```python
from build123d import *

# Parameters (mm, degrees)
EXTRUDE_1_DEPTH     = 3
EXTRUDE_2_DEPTH     = 51
EXTRUDE_3_DEPTH     = 3
FILLET_1_R          = 2
CHAMFER_1_SIZE      = 0.5
SKETCH_4_W          = 10
SKETCH_4_H          = 38
CUT_EXTRUDE_1_DEPTH = 59.180882402
FILLET_2_R          = 3


with BuildPart() as part:
    # 草图1 → 凸台-拉伸1 (new body)
    with BuildSketch(Plane.XY):
        with BuildLine():
            Line((-4, 1.5), (4, 1.5))
            ThreePointArc((4, 1.5), (5.5, 0), (4, -1.5))
            Line((4, -1.5), (-4, -1.5))
            ThreePointArc((-4, -1.5), (-5.5, 0), (-4, 1.5))
        make_face()
    extrude(amount=EXTRUDE_1_DEPTH)

    # 草图2 → 凸台-拉伸2 (add)
    with BuildSketch(Plane.XY.offset(3)):
        with BuildLine():
            Line((-10, 4.501256289), (-10, -1.5))
            Line((-10, -1.5), (-4, -1.5))
            ThreePointArc((-4, -1.5), (-5.5, 0), (-4, 1.5))
            Line((-4, 1.5), (4, 1.5))
            ThreePointArc((4, 1.5), (5.5, 0), (4, -1.5))
            Line((4, -1.5), (10, -1.5))
            Line((10, -1.5), (10, 4.501256289))
            ThreePointArc((10, 4.501256289), (0, 4), (-10, 4.501256289))
        make_face()
        with BuildLine():
            Line((4, 1.5), (-4, 1.5))
            ThreePointArc((-4, 1.5), (-5.5, 0), (-4, -1.5))
            Line((-4, -1.5), (4, -1.5))
            ThreePointArc((4, -1.5), (5.5, 0), (4, 1.5))
        make_face()
    extrude(amount=EXTRUDE_2_DEPTH)

    # 草图3 → 凸台-拉伸3 (add)
    with BuildSketch(Plane.XY.offset(54)):
        with BuildLine():
            Line((-3.954732622, 1.5), (4.045267378, 1.5))
            ThreePointArc((4.045267378, 1.5), (5.545267378, 0), (4.045267378, -1.5))
            Line((4.045267378, -1.5), (-3.954732622, -1.5))
            ThreePointArc((-3.954732622, -1.5), (-5.454732622, 0), (-3.954732622, 1.5))
        make_face()
    extrude(amount=EXTRUDE_3_DEPTH)

    # 圆角1
    fillet_1_edges = [part.edges().sort_by_distance(p)[0] for p in [
        (-10, -1.5, 28.5),
        (10, -1.5, 28.5),
    ]]
    fillet(fillet_1_edges, radius=FILLET_1_R)

    # 倒角1
    chamfer_1_edges = [part.edges().sort_by_distance(p)[0] for p in [
        (-5.454732622, 0, 57),
        (0.045267378, -1.5, 57),
        (5.545267378, 0, 57),
        (0.045267378, 1.5, 57),
        (0, 1.5, 0),
        (5.5, 0, 0),
        (0, -1.5, 0),
        (-5.5, 0, 0),
    ]]
    chamfer(chamfer_1_edges, length=CHAMFER_1_SIZE)

    # 草图4 → 切除-拉伸1 (cut, through all)
    with BuildSketch(Plane.XZ.offset(1.5)):
        with Locations((0, 28)):
            Rectangle(SKETCH_4_W, SKETCH_4_H)
    extrude(amount=-CUT_EXTRUDE_1_DEPTH, mode=Mode.SUBTRACT)

    # 圆角2
    fillet_2_edges = [part.edges().sort_by_distance(p)[0] for p in [
        (5, 1.312539111, 47),
        (5, 1.312539111, 9),
        (-5, 1.312539111, 9),
        (-5, 1.312539111, 47),
    ]]
    fillet(fillet_2_edges, radius=FILLET_2_R)


solid = part.part
```
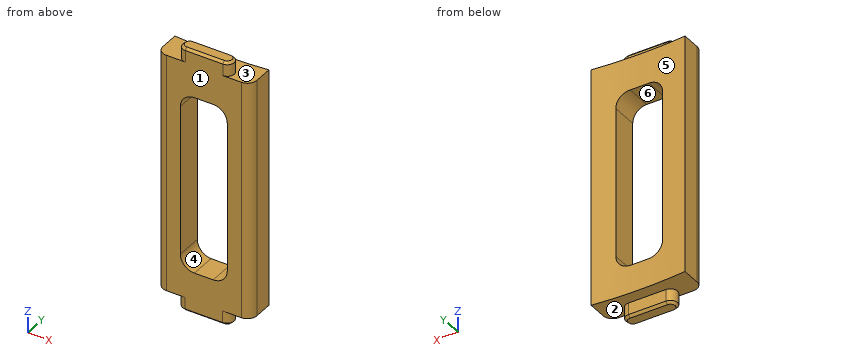
The listing builds one solid part. Answer for the finished solid, in the listing's coordinates (mm). Face numbers are marked on the shaded views. A direction names the side the tool comes from. Give positions to 0.01 mm unless a question says otherwise; leave off trailing zeros. Order: outer loops, then holes, each group sorted by start corner. A loop starts at its lowest first (then second) coordinate and runs counter-clockwise, first axis right, second up. Notation, with made-up numbers: (9.5, 1.5) - (27.5, 1.5) arc R21 ccw to (27.5, 37.5) - close; hole circle Ø7 at (38, -0.75). An arc over 180 degrees is marked (long way). Answer in a Markdown table with one row per item. Add a question column.
Q1. The part is cut by section C-C (z = 5.5). Determine the outline of the cut face in (x, y).
Q2. Find the intervals of material crossed by line 1 along X through (y, z) = (3.5, 27); line 2 along Z through (x, y) = (-0.25, 1); line 3 along Z through (x, y) = (-2, 3.5), in increasing order. Write a range as [from, to].
Q3. The part is cut by section B-B (y = 2). Determine the outline of the cut face in (x, z).
Q4. For a pull along Z with two mould halves and no side action, classify the marked faces 1, 2, 3 and 4 as released by +Z, released by -Z, zero draft, split by the parting line, or undercut.
Q5. The part is cut by section D-D (x = -7.5). Determine the outline of the cut face in (y, z), then the cut area to 3 significant figures.
Q6. Which of the six approach directions +Z, -Z, +X, -X, +Y, -Y give full straight-line access (tool end or side, diameter ignored) to the marked faces 5 and 6?
Q7. Given P1, Ø12, axis at x = 2, z = 39, coming from the +Y side; P2, Ø2, axis at x = 0.5, z = 1.5, coming from the +Y side; P3, Ø5, axis at x = -6, z = 33.5, coming from the +Y side, each flat-ended and moving along its own axis, determine where each tip first touches the part or whether it passes through.
Q8. The part is cut by section A-A (z = 43.5). Determine the outline of the cut face in (x, y).
Determined:
| question | item | result |
|---|---|---|
| 1 | outline | (-10, 0.5) arc R2 ccw to (-8, -1.5) - (8, -1.5) arc R2 ccw to (10, 0.5) - (10, 4.5) arc R100 cw to (-10, 4.5) - close |
| 2 | line 1 | x = [-10, -5], [5, 10] |
| 2 | line 2 | z = [0, 9], [47, 57] |
| 2 | line 3 | z = [3, 9], [47, 54] |
| 3 | outline | (-10, 3) - (10, 3) - (10, 54) - (-10, 54) - close; hole (-5, 12) arc R3 ccw to (-2, 9) - (2, 9) arc R3 ccw to (5, 12) - (5, 44) arc R3 ccw to (2, 47) - (-2, 47) arc R3 ccw to (-5, 44) - close |
| 4 | face 1 | zero draft |
| 4 | face 2 | released by -Z |
| 4 | face 3 | released by +Z |
| 4 | face 4 | undercut |
| 5 | outline | (-1.5, 3) - (4.28, 3) - (4.28, 54) - (-1.5, 54) - close |
| 5 | area | 295 mm² |
| 6 | face 5 | +Z, -Z, +Y |
| 6 | face 6 | +Y, -Y |
| 7 | P1 | stops at y = 4.32 |
| 7 | P2 | stops at y = 1.5 |
| 7 | P3 | stops at y = 4.36 |
| 8 | outline | (-10, 0.5) arc R2 ccw to (-8, -1.5) - (-5, -1.5) - (-5, 4.13) arc R100 cw to (-10, 4.5) - close; (5, -1.5) - (8, -1.5) arc R2 ccw to (10, 0.5) - (10, 4.5) arc R100 cw to (5, 4.13) - close |
